from build123d import *

# Parameters (mm, degrees)
SKETCH1_W           = 55
SKETCH1_H           = 30
BOSS_EXTRUDE1_DEPTH = 3
SKETCH2_W           = 7
SKETCH2_H           = 30
BOSS_EXTRUDE2_DEPTH = 30
SKETCH3_R           = 2.75
CUT_EXTRUDE1_DEPTH  = 10
CUT_EXTRUDE2_REACH  = 57
CUT_EXTRUDE3_REACH  = 35
SKETCH5_R           = 5


with BuildPart() as part:
    # Sketch1 → Boss-Extrude1 (new body)
    with BuildSketch(Plane(origin=(0, 0, 0), x_dir=(1, 0, 0), z_dir=(0, 1, 0))):
        Rectangle(SKETCH1_W, SKETCH1_H)
    extrude(amount=BOSS_EXTRUDE1_DEPTH)

    # Sketch2 → Boss-Extrude2 (add)
    with BuildSketch(Plane(origin=(0, 3, 0), x_dir=(1, 0, 0), z_dir=(0, 1, 0))):
        Polygon((-27.5, -12), (-27.5, -15), (-20.5, -15), (-20.5, 15), (-27.5, 15), align=None)
        with Locations((24, 0)):
            Rectangle(SKETCH2_W, SKETCH2_H)
    extrude(amount=BOSS_EXTRUDE2_DEPTH)

    # Sketch3 → Cut-Extrude1 (cut)
    with BuildSketch(Plane(origin=(0, 33, 0), x_dir=(1, 0, 0), z_dir=(0, 1, 0))):
        with Locations((-24, 5.5)):
            Circle(SKETCH3_R)
        with Locations((-24, -5.5)):
            Circle(SKETCH3_R)
        with Locations((24, -5.5)):
            Circle(SKETCH3_R)
        with Locations((24, 5.5)):
            Circle(SKETCH3_R)
    extrude(amount=-CUT_EXTRUDE1_DEPTH, mode=Mode.SUBTRACT)

    # Sketch4 → Cut-Extrude2 (cut, up to next)
    with BuildSketch(Plane.ZY.offset(27.5), mode=Mode.PRIVATE) as cut_extrude2_sk1:
        with BuildLine():
            Line((3.5, 22), (3.5, 7))
            ThreePointArc((3.5, 7), (0, 3.5), (-3.5, 7))
            Line((-3.5, 7), (-3.5, 22))
            ThreePointArc((-3.5, 22), (0, 25.5), (3.5, 22))
        make_face()
    cut_extrude2_tool1 = extrude(cut_extrude2_sk1.sketch, amount=-CUT_EXTRUDE2_REACH, mode=Mode.PRIVATE) & part.part
    add(cut_extrude2_tool1.solids().sort_by_distance((-27.5, 14.5, 0))[0], mode=Mode.SUBTRACT)

    # Sketch5 → Cut-Extrude3 (cut, up to next)
    with BuildSketch(Plane.XZ, mode=Mode.PRIVATE) as cut_extrude3_sk1:
        with Locations((-10, 0)):
            Circle(SKETCH5_R)
    cut_extrude3_tool1 = extrude(cut_extrude3_sk1.sketch, amount=-CUT_EXTRUDE3_REACH, mode=Mode.PRIVATE) & part.part
    add(cut_extrude3_tool1.solids().sort_by_distance((-10, 0, 0))[0], mode=Mode.SUBTRACT)


solid = part.part
Here's how the part is built. I have some questions about the finished solid (model axes, mm). A direction names the side the tool comes from. Give positions to 0.01 mm unless a question says otherwise; leave off trailing zeros. Loops run counter-clockwise (first coordinate to the right, second up) from the corner with the lowest first, then second, coordinate; pieces in that order, holes last. Notation, with made-up numbers: (-2.5, 78) -> (35.5, 78) arc R32 ccw to (35.5, 117) -> close; hole circle Ø3 at (-1.5, 1). An arc over 180 degrees is marked (long way). One line per item, written item: value.
Q1. Suppose I cut it at C-C on z = 0. Please give me the cut outline in (x, y), then the cut area to 3 significant figures.
Answers follow:
outline: (-27.5, 0) -> (-15, 0) -> (-15, 3) -> (-20.5, 3) -> (-20.5, 3.5) -> (-27.5, 3.5) -> close; (-27.5, 25.5) -> (-20.5, 25.5) -> (-20.5, 33) -> (-27.5, 33) -> close; (-5, 0) -> (27.5, 0) -> (27.5, 33) -> (20.5, 33) -> (20.5, 3) -> (-5, 3) -> close
area: 401 mm^2
Q2. Suppose I cut it at B-B on x = -10. Please give me the cut outline in (y, z).
Answers follow:
outline: (0, -15) -> (3, -15) -> (3, -5) -> (0, -5) -> close; (0, 5) -> (3, 5) -> (3, 15) -> (0, 15) -> close
Q3. I'm going to push flat-ended pins straight in: pin 1 Ø5 at (x, z) = (24, -5.5) entering from -Y; pin 2 Ø4 at (x, z) = (-3.5, -7.5) entering from +Y; pin 3 Ø4 at (x, z) = (-24.5, 5) entering from +Y. Where does each tip first touch, or does it pass through?
Answers follow:
pin 1: y = 0
pin 2: y = 3
pin 3: y = 23
Q4. Suppose I cut it at D-D on z = -11.5. Please give me the cut outline in (x, y).
Answers follow:
outline: (-27.5, 0) -> (27.5, 0) -> (27.5, 33) -> (20.5, 33) -> (20.5, 3) -> (-20.5, 3) -> (-20.5, 33) -> (-27.5, 33) -> close
Q5. Suppose I cut it at A-A on y = 17. Please give me the cut outline in (x, z).
Answers follow:
outline: (-27.5, -15) -> (-20.5, -15) -> (-20.5, -3.5) -> (-27.5, -3.5) -> close; (-27.5, 3.5) -> (-20.5, 3.5) -> (-20.5, 15) -> (-27.5, 15) -> close; (20.5, -15) -> (27.5, -15) -> (27.5, 15) -> (20.5, 15) -> close
Q6. We'd pull the mould along Y, two halves only. Please class faces 4 (the face through (-24, 25.5, -0.1)), 5 (the face through (-24, 33, 0)), 6 (the face through (-24, 3.5, 0.1)), 7 (the face through (27.5, 16, 0)): pulls with the +Y half, pulls with the -Y half, needs draft (parallel to the pull), parting line crosses it, or undercut.
Answers follow:
face 4: undercut
face 5: pulls with the +Y half
face 6: undercut
face 7: needs draft
Q7. If I drill on line 1 along Z through (x, y) = (-24, 29); line 2 along X through (y, z) = (30, 5.5); line 3 along X through (y, z) = (4, -8.75), over which ranges is the centre line in solid material (lowest first)?
Answers follow:
line 1: -15 to -8.25, -2.75 to 2.75, 8.25 to 15
line 2: -27.5 to -26.75, -21.25 to -20.5, 20.5 to 21.25, 26.75 to 27.5
line 3: -27.5 to -20.5, 20.5 to 27.5
Q8. On a 3-axis mill with a long thin cutter (end or side, diameter ignored), from which of +Z, -Z, +X, -X, +Y, -Y can I reach the whole of each face in a straight line? I mean faces 1 (the face through (-24, 15, 3.5)), 2 (the face through (24, 23, 5)), 3 (the face through (-20.5, 18, 4)). Say none if no direction works.
Answers follow:
face 1: -X
face 2: +Y
face 3: +Z, -Z, +Y
